```python
from build123d import *

# Parameters (mm, degrees)
CYLINDER006_R     = 3.5
CYLINDER006_DEPTH = 10
CYLINDER005_R     = 1.65
CYLINDER005_DEPTH = 31
CYLINDER001_R     = 2.525
CYLINDER001_DEPTH = 35
CYLINDER009_R     = 3.1
CYLINDER009_DEPTH = 19
BOX013_W          = 7.8
BOX013_H          = 15
BOX013_DEPTH      = 1
BOX015_W          = 8
BOX015_H          = 20
BOX015_DEPTH      = 12
CHAMFER007_SIZE   = 5
FILLET001_R       = 1
FILLET_R          = 1
BOX009_W          = 7
BOX009_H          = 7.8
BOX009_DEPTH      = 8
CHAMFER006_SIZE   = 0.4
BOX010_W          = 18
BOX010_H          = 42
BOX010_DEPTH      = 8
CHAMFER008_SIZE   = 7
CHAMFER009_SIZE   = 10
FILLET003_R       = 1
BOX011_W          = 27
BOX011_H          = 15
BOX011_DEPTH      = 10
FILLET004_R       = 3


with BuildPart() as cylinder006:
    # Cylinder006 → Cylinder006 (new body)
    with BuildSketch(Plane(origin=(9, 34, 37), x_dir=(1, 0, 0), z_dir=(0, 0, 1))):
        Circle(CYLINDER006_R)
    extrude(amount=CYLINDER006_DEPTH)


with BuildPart() as fusion009:
    # Cylinder005 → Cylinder005 (new body)
    with BuildSketch(Plane(origin=(9, 34, 19), x_dir=(1, 0, 0), z_dir=(0, 0, 1))):
        Circle(CYLINDER005_R)
    extrude(amount=CYLINDER005_DEPTH)

    # Fusion009: union Cylinder006
    add(cylinder006.part)


with BuildPart() as cylinder001:
    # Cylinder001 → Cylinder001 (new body)
    with BuildSketch(Plane(origin=(9, 15, 5), x_dir=(1, 0, 0), z_dir=(0, 0, 1))):
        Circle(CYLINDER001_R)
    extrude(amount=CYLINDER001_DEPTH)


with BuildPart() as cylinder009:
    # Cylinder009 → Cylinder009 (new body)
    with BuildSketch(Plane(origin=(-15, 37.5, 25), x_dir=(1, 0, 0), z_dir=(0, 0, 1))):
        Circle(CYLINDER009_R)
    extrude(amount=CYLINDER009_DEPTH)


with BuildPart() as cube013:
    # Box013 → Box013 (new body)
    with BuildSketch(Plane(origin=(-18.9, 30, 29), x_dir=(1, 0, 0), z_dir=(0, 0, 1))):
        with Locations((3.9, 7.5)):
            Rectangle(BOX013_W, BOX013_H)
    extrude(amount=BOX013_DEPTH)


with BuildPart() as fillet_body:
    # Box015 → Box015 (new body)
    with BuildSketch(Plane(origin=(7, 25, 20), x_dir=(1, 0, 0), z_dir=(0, 0, 1))):
        with Locations((4, 10)):
            Rectangle(BOX015_W, BOX015_H)
    extrude(amount=BOX015_DEPTH)

    # Chamfer007
    chamfer007_edges = [fillet_body.edges().sort_by_distance(p)[0] for p in [
        (15, 45, 26),
    ]]
    chamfer(chamfer007_edges, length=CHAMFER007_SIZE)

    # Fillet001
    fillet001_edges = [fillet_body.edges().sort_by_distance(p)[0] for p in [
        (15, 40, 26),
        (15, 25, 26),
        (7, 25, 26),
        (7, 45, 26),
    ]]
    fillet(fillet001_edges, radius=FILLET001_R)


with BuildPart() as fillet_body_1:
    # Fillet001 placement: moved
    add(fillet_body.part.moved(Location((-2, 0, 0))))

    # Fillet
    fillet_edges = [fillet_body_1.edges().sort_by_distance(p)[0] for p in [
        (8, 45, 26),
    ]]
    fillet(fillet_edges, radius=FILLET_R)


with BuildPart() as chamfer006:
    # Box009 → Box009 (new body)
    with BuildSketch(Plane(origin=(-7, 11.1, 32), x_dir=(1, 0, 0), z_dir=(0, 0, 1))):
        with Locations((3.5, 3.9)):
            Rectangle(BOX009_W, BOX009_H)
    extrude(amount=BOX009_DEPTH)

    # Chamfer006
    chamfer006_edges = [chamfer006.edges().sort_by_distance(p)[0] for p in [
        (-7, 11.1, 36),
        (-7, 18.9, 36),
    ]]
    chamfer(chamfer006_edges, length=CHAMFER006_SIZE)


with BuildPart() as fillet003:
    # Box010 → Box010 (new body)
    with BuildSketch(Plane(origin=(0, 3, 32), x_dir=(1, 0, 0), z_dir=(0, 0, 1))):
        with Locations((9, 21)):
            Rectangle(BOX010_W, BOX010_H)
    extrude(amount=BOX010_DEPTH)

    # Chamfer008
    chamfer008_edges = [fillet003.edges().sort_by_distance(p)[0] for p in [
        (18, 3, 36),
    ]]
    chamfer(chamfer008_edges, length=CHAMFER008_SIZE)

    # Chamfer009
    chamfer009_edges = [fillet003.edges().sort_by_distance(p)[0] for p in [
        (18, 45, 36),
    ]]
    chamfer(chamfer009_edges, length=CHAMFER009_SIZE)

    # Fillet003
    fillet003_edges = [fillet003.edges().sort_by_distance(p)[0] for p in [
        (18, 35, 36),
        (18, 10, 36),
        (8, 45, 36),
        (11, 3, 36),
    ]]
    fillet(fillet003_edges, radius=FILLET003_R)


with BuildPart() as cut002002002009004:
    # Box011 → Box011 (new body)
    with BuildSketch(Plane(origin=(-27, 30, 30), x_dir=(1, 0, 0), z_dir=(0, 0, 1))):
        with Locations((13.5, 7.5)):
            Rectangle(BOX011_W, BOX011_H)
    extrude(amount=BOX011_DEPTH)

    # Fillet004
    fillet004_edges = [cut002002002009004.edges().sort_by_distance(p)[0] for p in [
        (-27, 30, 35),
        (-27, 45, 35),
    ]]
    fillet(fillet004_edges, radius=FILLET004_R)

    # Fusion010: union Cube013, Fillet body, Chamfer006, Fillet003
    add(cube013.part)
    add(fillet_body_1.part)
    add(chamfer006.part)
    add(fillet003.part)

    # Cut002002002009002: cut Cylinder009
    add(cylinder009.part, mode=Mode.SUBTRACT)

    # Cut002002002009003: cut Cylinder001
    add(cylinder001.part, mode=Mode.SUBTRACT)

    # Cut002002002009004: cut Fusion009
    add(fusion009.part, mode=Mode.SUBTRACT)


solid = cut002002002009004.part
```
For this review, take the finished solid that the model builds, in its own axes (mm). A direction names the side the tool comes from. Round coordinates to 2 decimals unless told otherwise and drop trailing zeros. Loops run counter-clockwise (first coordinate to the right, second up) from the corner with the lowest first, then second, coordinate; pieces in that order, holes last.
(1) We need section D-D (y = 23). Give the boundary of the cut face in (x, z), plus the area to 3 significant figures.
Returned:
outline: (0, 32) - (18, 32) - (18, 40) - (0, 40) - close
area: 144 mm2
(2) Clearance check with flat-ended pins moving along their axes: P1, Ø6, axis at y = 36, z = 24, coming from the -X side; P2, Ø9, axis at x = -6, y = 39.5, coming from the -Z side; P3, Ø4, axis at y = 36.5, z = 26, coming from the +X side. State where each tip first meets the part, or that it passes through.
Returned:
P1: stops at x = 5
P2: stops at z = 30
P3: stops at x = 13
(3) Wall thickness on line 1 along Y through (x, z) = (9, 37.75) (3 decimals); line 2 along Y through (x, z) = (9, 34) (3 decimals); line 3 along X through (y, z) = (34, 29.25): over which ranges is each line inside the solid? List them lowest first.
Returned:
line 1: y = 3 to 12.475, 17.525 to 30.5, 37.5 to 44
line 2: y = 3 to 12.475, 17.525 to 32.35, 35.65 to 44
line 3: x = -18.9 to -11.1, 5 to 7.35, 10.65 to 13
(4) We need section C-C (x = -15). Give the boundary of the cut face in (y, z), plus the area to 3 significant figures.
Returned:
outline: (30, 29) - (34.4, 29) - (34.4, 40) - (30, 40) - close; (40.6, 29) - (45, 29) - (45, 40) - (40.6, 40) - close
area: 96.8 mm2
(5) We need section A-A (x = 9). Give the boundary of the cut face in (y, z) (3 decimals), plus the area to 4 significant figures.
Returned:
outline: (3, 32) - (12.475, 32) - (12.475, 40) - (3, 40) - close; (17.525, 32) - (25, 32) - (25, 20) - (32.35, 20) - (32.35, 37) - (30.5, 37) - (30.5, 40) - (17.525, 40) - close; (35.65, 20) - (44, 20) - (44, 40) - (37.5, 40) - (37.5, 37) - (35.65, 37) - close
area: 438.5 mm2
(6) We need section B-B (y = 15). Give the boundary of the cut face in (x, z) (3 decimals).
Returned:
outline: (-7, 32) - (6.475, 32) - (6.475, 40) - (-7, 40) - close; (11.525, 32) - (18, 32) - (18, 40) - (11.525, 40) - close
(7) Mouldability with a two-part tool opening along X and no side actions: class faces 1 (the flat face through (15, 7, 36)), 2 (the cylindrical face through (-26.14, 30.9, 35.07)), 3 (the cylindrical face through (8.671, 17.504, 35.944)), 4 (the cylindrical face through (5.301, 44.715, 26.084)) as released by +X, released by -X, zero draft, split by the parting line, or undercut.
Returned:
face 1: released by +X
face 2: released by -X
face 3: undercut
face 4: undercut
(8) Tool access review of faces 5 (the flat face through (-3, 18.9, 36)), 6 (the flat face through (-18, 39, 29)), 7 (the flat face through (-7, 15, 36)): name each direction out of +Z, -Z, +X, -X, +Y, -Y from which nothing blocks a thin tool from reaching the whole face with its end or side.
Returned:
face 5: +Z, -Z, -X
face 6: -Z, -X, +Y, -Y
face 7: +Z, -Z, -X, -Y
